The model under review builds one solid part; all positions refer to its coordinate system, in mm. A direction names the side the tool comes from. Give positions to 0.01 mm unless a question says otherwise; leave off trailing zeros. Loops run counter-clockwise (first coordinate to the right, second up) from the corner with the lowest first, then second, coordinate; pieces in that order, holes last. Notation, with made-up numbers: (14, -6) -> (47, -6) arc R21 cw to (47, 7) -> close; hole circle Ø1 at (38, -24). An arc over 180 degrees is marked (long way). Write each question's results on one line, items separated by ' | '. Start each with the question number.
Q1. We need section B-B (y = 3.5). Write out the cut boundary in (x, z) (3 decimals).
Q2. Insertion check: pin 1 Ø4 at (x, z) = (-2.5, 2.5) entering from +Y; pin 2 Ø3 at (x, z) = (1.5, 2) entering from +Y; pin 3 Ø1.1 at (x, z) = (-0.5, -4.5) entering from +Y. Each pin has a flat end and moves straight along its axis. Give the tip position at first contact, or say it passes through.
Q3. Machinability: for faces 1 (the face through (4, 1.588, 3)), 2 (the face through (2.9, 1.97, 3.78)), 3 (the face through (-4.3, 0, -2.4)), 4 (the face through (4.3, 1.588, -2.4)), 5 (the face through (-4.3, 1.588, -2.4)), which of the approach directions +Z, -Z, +X, -X, +Y, -Y give a long, thin tool a straight path to every point of the face, cutting with its end or side? Answer none if there is none.
Q4. Wall thickness on L1, parallel to X at y = -0.1, z = 0 (1 decimal); L2, parallel to Z at x = -1.5, y = 2: over which ranges is each line inside the solid? List them lowest first. Write a range as [from, to].
from build123d import *

# Parameters (mm, degrees)
SKETCH1_R           = 3.175
BOSS_EXTRUDE1_DEPTH = 1.5875
SKETCH2_W           = 1.5875
SKETCH2_H           = 0.254


with BuildPart() as part:
    # Sketch1 → Boss-Extrude1 (new body)
    with BuildSketch(Plane(origin=(0, 0, 0), x_dir=(1, 0, 0), z_dir=(0, 1, 0))):
        Polygon((4.7625, 2.749630657), (0, 5.499261314), (-4.7625, 2.749630657), (-4.7625, -2.749630657), (0, -5.499261314), (4.7625, -2.749630657), align=None)
        Circle(SKETCH1_R, mode=Mode.SUBTRACT)
    extrude(amount=BOSS_EXTRUDE1_DEPTH)

    # Sketch2 → Revolve1 (revolve)
    with BuildSketch(Plane(origin=(0, 0, 0), x_dir=(0, 0, -1), z_dir=(1, 0, 0))):
        with BuildLine():
            Line((3.6576, 3.2004), (3.6576, 4.2926))
            ThreePointArc((3.6576, 4.2926), (2.586313763, 6.878913763), (0, 7.9502))
            Line((0, 7.9502), (0, 7.4676))
            ThreePointArc((0, 7.4676), (2.24506403, 6.53766403), (3.175, 4.2926))
            Line((3.175, 4.2926), (3.175, 1.5875))
            Line((3.175, 1.5875), (4.7625, 1.5875))
            Line((4.7625, 1.5875), (4.7625, 2.3495))
            Line((4.7625, 2.3495), (4.5085, 2.3495))
            Line((4.5085, 2.3495), (3.6576, 3.2004))
        make_face()
        with Locations((3.96875, -0.127)):
            Rectangle(SKETCH2_W, SKETCH2_H)
    revolve(axis=Axis((0, 0, 0), (0, 1, 0)))


solid = part.part
Output:
1) outline: circle Ø7.315 at (0, 0); hole circle Ø6.35 at (0, 0)
2) pin 1: y = 7.61 | pin 2: y = 7.81 | pin 3: y = 2.88
3) face 1: +Z, +X, +Y | face 2: +Y | face 3: -Z, -X, -Y | face 4: -Z, +X, +Y | face 5: -Z, -X, +Y
4) L1: [-4.8, -3.2], [3.2, 4.8] | L2: [-4.52, -2.8], [2.8, 4.52]
